CAD build for the part. Positions are in the model's coordinates, mm. Face numbers are marked on the shaded views. A direction names the side the tool comes from. Round coordinates to 2 decimals unless told otherwise and drop trailing zeros. Write each loop counter-clockwise with the first axis right and the second up, starting at its lowest first coordinate (ties: lowest second). Pieces come first, ordered by that corner, then holes. Notation, with made-up numbers: (64, -21) -> (99, -21) arc R25 ccw to (99, 15) -> close; hole circle Ø2 at (-11, 21). An arc over 180 degrees is marked (long way). Put each result on its own line as item: value. Start each with the question number.
1. Saw through at A-A on y = -3. List the corners of the cut face in (x, z), and give its area (3 significant figures).
2. 3-axis set-ups, long thin cutter, end or side, ignore diameter. For the marked faces 1 and 2: which of +Z, -Z, +X, -X, +Y, -Y reach the whole face in a straight line?
3. Pull direction Z, two halves, no side cores. Call the marked faces 3, 4, 5 and 6: pulls with the +Z half, pulls with the -Z half, needs draft (parallel to the pull), parting line crosses it, or undercut.
4. Saw through at B-B on x = 26.5. List the corners of the cut face in (y, z).
5. Saw through at C-C on z = 5.25. List the corners of the cut face in (x, y), and give its area (3 significant figures).
6. Flat gauge pin, fed straight in: P1, Ø3, axis at y = -8, z = 8, coming from the -X side. Where does the tip first touch, or does it go through?
7. Drill centre lines: line 1 (Z direction, x = -29, y = 7); line 2 (X direction, y = -1.5, z = 11.5). Where is each one in solid material? Low to high. Write a range as from..to.
from build123d import *

# Parameters (mm, degrees)
SKETCH1_W           = 25.4
SKETCH1_H           = 25.4
BOSS_EXTRUDE1_DEPTH = 114.3
CUT_EXTRUDE1_DEPTH  = 685.8
SKETCH5_W           = 22.098
SKETCH5_H           = 22.098
CUT_EXTRUDE3_DEPTH  = 230.304470083
CUT_EXTRUDE4_DEPTH  = 685.8


with BuildPart() as part:
    # Sketch1 → Boss-Extrude1 (new, symmetric)
    with BuildSketch(Plane(origin=(0, 0, 0), x_dir=(0, 0, -1), z_dir=(1, 0, 0))):
        Rectangle(SKETCH1_W, SKETCH1_H)
    extrude(amount=BOSS_EXTRUDE1_DEPTH, both=True)

    # Sketch2 → Cut-Extrude1 (cut)
    with BuildSketch(Plane(origin=(0, 12.7, 0), x_dir=(1, 0, 0), z_dir=(0, 1, 0))):
        Polygon((114.3, -12.7), (101.358053583, 12.7), (114.3, 12.7), align=None)
    extrude(amount=-CUT_EXTRUDE1_DEPTH, mode=Mode.SUBTRACT)

    # Sketch5 → Cut-Extrude3 (cut, through all)
    with BuildSketch(Plane.ZY.offset(114.3)):
        Rectangle(SKETCH5_W, SKETCH5_H)
    extrude(amount=-CUT_EXTRUDE3_DEPTH, mode=Mode.SUBTRACT)

    # Sketch6 → Cut-Extrude4 (cut)
    with BuildSketch(Plane(origin=(0, 12.7, 0), x_dir=(1, 0, 0), z_dir=(0, 1, 0))):
        Polygon((-114.3, -12.7), (-101.358053583, 12.7), (-114.3, 12.7), align=None)
    extrude(amount=-CUT_EXTRUDE4_DEPTH, mode=Mode.SUBTRACT)


solid = part.part
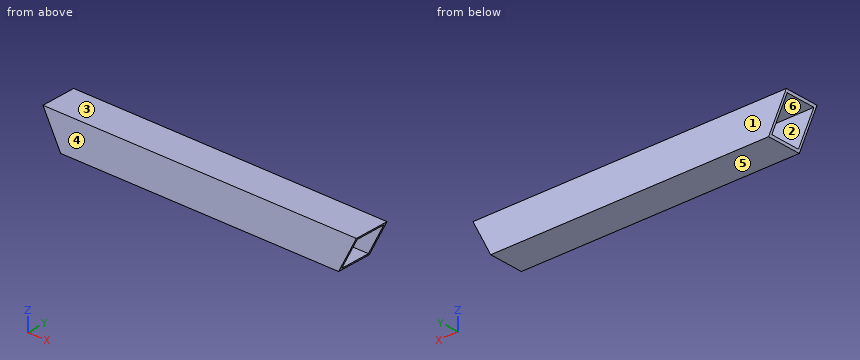
Return value:
1. outline: (-114.3, 12.7) -> (-113.46, 11.05) -> (113.46, 11.05) -> (114.3, 12.7) -> close; (-102.2, -11.05) -> (-101.36, -12.7) -> (101.36, -12.7) -> (102.2, -11.05) -> close
1. area: 712 mm^2
2. face 1: +Z, -Z, +X, -X, +Y
2. face 2: +X, -X
3. face 3: pulls with the +Z half
3. face 4: needs draft
3. face 5: pulls with the -Z half
3. face 6: undercut
4. outline: (-12.7, -12.7) -> (12.7, -12.7) -> (12.7, 12.7) -> (-12.7, 12.7) -> close; hole (-11.05, -11.05) -> (11.05, -11.05) -> (11.05, 11.05) -> (-11.05, 11.05) -> close
5. outline: (-110.5, -12.7) -> (110.5, -12.7) -> (110.5, -11.05) -> (-110.5, -11.05) -> close; (-110.5, 11.05) -> (110.5, 11.05) -> (110.5, 12.7) -> (-110.5, 12.7) -> close
5. area: 730 mm^2
6. P1: passes through
7. line 1: z = -12.7..-11.05, 11.05..12.7
7. line 2: x = -113.69..113.69
